Check sheet for the modelled part. Datum: model origin and axes. Units: mm. A direction names the side the tool comes from. Round coordinates to 2 decimals unless told otherwise and drop trailing zeros. Write item = value, one per line. Start each with the question number.
(1) Mould release check, pull along Z, two halves, no side actions. Record for faces 4 (the face through (27.371, 86.915, -9.051)), 5 (the face through (-89.3, -20.3, -10.616)), 6 (the face through (1, 1, 0)), 7 (the face through (-85.96, 51.12, 2.35)): pulls with the +Z half, pulls with the -Z half, needs draft (parallel to the pull), parting line crosses it, or undercut.
(2) Scan lines: L1, parallel to Z at x = -28.5, y = -87.5; L2, parallel to Y at x = -0.5, z = -10; L3, parallel to Y at x = -25.4, z = 2.25. Record each from-to range of solid material in increasing order. Write a range as from..to.
(3) Go/stop test with flat-tipped pins: P1, Ø4.5, axis at x = 0, y = 41.35, coming from the +Z side; P2, Ø1.5, axis at y = 62.5, z = -7.5, coming from the +X side; P3, Ø1.5, axis at x = 28, z = -6.5, coming from the +Y side; P4, Ø3, axis at x = -92.02, y = -53.13, coming from the +Z side. Record where each tip stops, or that it passes through.
(4) Set-up check for faces 1 (the face through (-89.34, 28.13, -6.2)), 2 (the face through (0.32, 108.692, 2.348)), 3 (the face through (-89.3, -20.3, -1.808)): record each of +Z, -Z, +X, -X, +Y, -Y from which the full face is reachable in a straight line by a thin tool's end or side.
from build123d import *

# Parameters (mm, degrees)
SKETCH1_R                        = 100.0125
EXTRUDE1_DEPTH                   = 4.7625
SKETCH2_R                        = 93.6625
EXTRUDE2_DEPTH                   = 12.7
SKETCH3_R                        = 87.3125
CUT_EXTRUDE1_DEPTH               = 12.7
SKETCH4_W                        = 3.175
SKETCH4_H                        = 2.54
EXTRUDE3_DEPTH                   = 4.7625
F_10_0_1935_DIAMETER_HOLE1_D     = 4.9149
F_10_0_1935_DIAMETER_HOLE1_DEPTH = 330.2
F_10_0_1935_DIAMETER_HOLE1_TIP   = 1.476584928
CHAMFER1_SIZE                    = 0.508
F_6_CLEARANCE_HOLE1_D            = 3.7973
F_6_CLEARANCE_HOLE1_DEPTH        = 6.35
F_6_CLEARANCE_HOLE1_TIP          = 1.140824014
F_6_CLEARANCE_HOLE2_D            = 3.7973
F_6_CLEARANCE_HOLE2_DEPTH        = 25.4
F_6_CLEARANCE_HOLE2_TIP          = 1.140824014


with BuildPart() as part:
    # Sketch1 → Extrude1 (new body)
    with BuildSketch(Plane.XY):
        Circle(SKETCH1_R)
    extrude(amount=EXTRUDE1_DEPTH)

    # Sketch2 → Extrude2 (add)
    with BuildSketch(Plane(origin=(0, 0, 0), x_dir=(-1, 0, 0), z_dir=(0, 0, -1))):
        Circle(SKETCH2_R)
    extrude(amount=EXTRUDE2_DEPTH)

    # Sketch3 → Cut-Extrude1 (cut)
    with BuildSketch(Plane(origin=(0, 0, -12.7), x_dir=(-1, 0, 0), z_dir=(0, 0, -1))):
        Circle(SKETCH3_R)
    extrude(amount=-CUT_EXTRUDE1_DEPTH, mode=Mode.SUBTRACT)

    # Sketch4 → Cut-Revolve1 (revolve, cut)
    with BuildSketch(Plane(origin=(0, 0, 0), x_dir=(0, 0, -1), z_dir=(1, 0, 0))):
        with Locations((3.395858926, 92.3925)):
            Rectangle(SKETCH4_W, SKETCH4_H)
        with Locations((9.028423409, 92.3925)):
            Rectangle(SKETCH4_W, SKETCH4_H)
    revolve(axis=Axis((0, 0, 0), (0, 0, -1)), mode=Mode.SUBTRACT)

    # Sketch5 → Extrude3 (add)
    with BuildSketch(Plane.XY.offset(4.7625)):
        with BuildLine():
            ThreePointArc((-12.674375762, 99.206150794), (0, 112.7125), (12.674375762, 99.206150794))
            ThreePointArc((12.674375762, 99.206150794), (0, 100.0125), (-12.674375762, 99.206150794))
        make_face()
        with BuildLine():
            ThreePointArc((92.25223468, -38.62674401), (97.611888324, -56.35625), (79.577858918, -60.579406784))
            ThreePointArc((79.577858918, -60.579406784), (86.613365696, -50.00625), (92.25223468, -38.62674401))
        make_face()
        with BuildLine():
            ThreePointArc((-79.577858918, -60.579406784), (-97.611888324, -56.35625), (-92.25223468, -38.62674401))
            ThreePointArc((-92.25223468, -38.62674401), (-86.613365696, -50.00625), (-79.577858918, -60.579406784))
        make_face()
    extrude(amount=-EXTRUDE3_DEPTH)

    # #10 (0.1935) Diameter Hole1
    with Locations(Plane(origin=(0, 106.25582337, 4.7625), x_dir=(1, 0, 0), z_dir=(0, 0, 1))):
        with Locations((0, 0), (-92.020242338, -159.383735055), (92.020242338, -159.383735055)):
            Hole(F_10_0_1935_DIAMETER_HOLE1_D / 2, depth=F_10_0_1935_DIAMETER_HOLE1_DEPTH)
            with Locations((0, 0, -(F_10_0_1935_DIAMETER_HOLE1_DEPTH + F_10_0_1935_DIAMETER_HOLE1_TIP / 2))):  # 118° drill point
                Cone(0, F_10_0_1935_DIAMETER_HOLE1_D / 2, F_10_0_1935_DIAMETER_HOLE1_TIP, mode=Mode.SUBTRACT)

    # Chamfer1
    chamfer1_edges = [part.edges().sort_by_distance(p)[0] for p in [
        (93.6625, 0, -1.808358926),
        (93.6625, 0, -4.983358926),
        (93.6625, 0, -7.440923409),
        (93.6625, 0, -10.615923409),
        (93.6625, 0, -12.7),
    ]]
    chamfer(chamfer1_edges, length=CHAMFER1_SIZE)

    # #6 Clearance Hole1
    with Locations(Plane(origin=(0, 63.952783211, 4.7625), x_dir=(1, 0, 0), z_dir=(0, 0, 1))):
        with Locations((0, 0), (0, -22.606), (0, -120.904)):
            Hole(F_6_CLEARANCE_HOLE1_D / 2, depth=F_6_CLEARANCE_HOLE1_DEPTH)
            with Locations((0, 0, -(F_6_CLEARANCE_HOLE1_DEPTH + F_6_CLEARANCE_HOLE1_TIP / 2))):  # 118° drill point
                Cone(0, F_6_CLEARANCE_HOLE1_D / 2, F_6_CLEARANCE_HOLE1_TIP, mode=Mode.SUBTRACT)

    # #6 Clearance Hole2
    with Locations(Plane(origin=(25.4, -57.15, 0), x_dir=(-1, 0, 0), z_dir=(0, 0, -1))):
        with Locations((0, 0), (50.8, 0), (0, -19.05), (50.8, -19.05)):
            Hole(F_6_CLEARANCE_HOLE2_D / 2, depth=F_6_CLEARANCE_HOLE2_DEPTH)
            with Locations((0, 0, -(F_6_CLEARANCE_HOLE2_DEPTH + F_6_CLEARANCE_HOLE2_TIP / 2))):  # 118° drill point
                Cone(0, F_6_CLEARANCE_HOLE2_D / 2, F_6_CLEARANCE_HOLE2_TIP, mode=Mode.SUBTRACT)


solid = part.part
Result:
q1.face_4 = undercut
q1.face_5 = undercut
q1.face_6 = pulls with the -Z half
q1.face_7 = needs draft
q2.L1 = -12.7..-10.62, -7.44..-4.98, -1.81..4.76
q2.L2 = -91.12..-87.31, 87.31..91.12
q2.L3 = -96.73..-78.1, -74.3..-59.05, -55.25..96.73
q3.P1 = 4.76
q3.P2 = 70.2
q3.P3 = 89.61
q3.P4 = through
q4.face_1 = -Z
q4.face_2 = +Z, -Z
q4.face_3 = none
